```python
from build123d import *

# Parameters (mm, degrees)
SKETCH_1_R      = 6.1
EXTRUDE_1_DEPTH = 4


with BuildPart() as part:
    # 스케치1 → 보스-돌출1 (new body)
    with BuildSketch(Plane.XY):
        with BuildLine():
            Line((-10.9, 20.333989173), (-10.9, -6.666010827))
            Line((-10.9, -6.666010827), (-8.65, -6.666010827))
            Line((-8.65, -6.666010827), (-6.9, -6.666010827))
            ThreePointArc((-6.9, -6.666010827), (0, 0.233989173), (6.9, -6.666010827))
            Line((6.9, -6.666010827), (8.65, -6.666010827))
            Line((8.65, -6.666010827), (10.9, -6.666010827))
            Line((10.9, -6.666010827), (10.9, 20.333989173))
            ThreePointArc((10.9, 20.333989173), (0, 31.233989173), (-10.9, 20.333989173))
        make_face()
        with Locations((0, 20.333989173)):
            Circle(SKETCH_1_R, mode=Mode.SUBTRACT)
    extrude(amount=EXTRUDE_1_DEPTH)


solid = part.part
```
Geometry: final body of the model. Coordinates: model frame, mm. Round coordinates to 2 decimals unless told otherwise and drop trailing zeros. Write each loop counter-clockwise with the first axis right and the second up, starting at its lowest first coordinate (ties: lowest second). Pieces come first, ordered by that corner, then holes. Notation, with made-up numbers: (-35.75, -9) -> (-31.75, -9) arc R16 ccw to (-31.75, 11) -> close; hole circle Ø9 at (29, -9.75). An arc over 180 degrees is marked (long way). Return JSON: item names as keys, results as strings.
Q1. Section B-B on z = 2.1. Return the cut outline in (x, y).
From the geometry:
{"outline": "(-10.9, -6.67) -> (-6.9, -6.67) arc R6.9 cw to (6.9, -6.67) -> (10.9, -6.67) -> (10.9, 20.33) arc R10.9 ccw to (-10.9, 20.33) -> close; hole circle Ø12.2 at (0, 20.33)"}
Q2. Section A-A on x = 0. Return the cut outline in (y, z).
From the geometry:
{"outline": "(0.23, 0) -> (14.23, 0) -> (14.23, 4) -> (0.23, 4) -> close; (26.43, 0) -> (31.23, 0) -> (31.23, 4) -> (26.43, 4) -> close"}
Q3. First-contact query: pin 1 Ø1 at (x, z) = (2.5, 3.5) entering from +Y; pin 2 Ø10 at (x, y) = (0, 20.33) entering from -Z. Flat tips, straight axial feed; report the tip coordinate or a pass-through.
From the geometry:
{"pin 1": "y = 31.05", "pin 2": "through"}
Q4. Ray query, line 1 (Y direction, x = 0, z = 2.6); line 2 (X direction, y = -4.5, z = 1.9); line 3 (X direction, y = 19.5, z = 0.4). Return the intervals inside material, ascending.
From the geometry:
{"line 1": "0.23 to 14.23, 26.43 to 31.23", "line 2": "-10.9 to -6.55, 6.55 to 10.9", "line 3": "-10.9 to -6.04, 6.04 to 10.9"}
Q5. Section D-D on y = 27. Return the cut outline in (x, z), and give its area (3 significant figures).
From the geometry:
{"outline": "(-8.62, 0) -> (8.62, 0) -> (8.62, 4) -> (-8.62, 4) -> close", "area": "69.0 mm2"}
Q6. Mould query, pull axis X, two halves, no side actions, for faces 1 (the flat face through (0, 13, 0)), 2 (the cylindrical face through (0.24, 31.23, 1.97)), 3 (the cylindrical face through (-4.84, 16.62, 1.97)). Classes: +X half, -X half, draft (parallel to the pull), parting line (faces both ways), or undercut.
From the geometry:
{"face 1": "draft", "face 2": "parting line", "face 3": "undercut"}
Q7. Section C-C on y = 21.5. Return the cut outline in (x, z).
From the geometry:
{"outline": "(-10.84, 0) -> (-5.99, 0) -> (-5.99, 4) -> (-10.84, 4) -> close; (5.99, 0) -> (10.84, 0) -> (10.84, 4) -> (5.99, 4) -> close"}
